The model under review builds one solid part; all positions refer to its coordinate system, in mm. Face numbers are marked on the shaded views. Round coordinates to 2 decimals unless told otherwise and drop trailing zeros. Order: outer loops, then holes, each group sorted by start corner. A loop starts at its lowest first (then second) coordinate and runs counter-clockwise, first axis right, second up. Notation, with made-up numbers: (22, 89.25) - (80, 89.25) arc R21 cw to (80, 106.25) - close; hole circle Ø7 at (4.5, 69.25). An arc over 180 degrees is marked (long way). One line per question, with ' | ' between items. Start each with the question number.
Item 1: For L1, parallel to X at y = 22, z = 5.25; L2, parallel to Y at x = -51, z = 15; L3, parallel to Z at x = -78.5, y = 29, list the stretches that pass through material, from the lowest coordinate up. Write a range as [from, to].
Item 2: Insertion check: pin 1 Ø2 at (x, y) = (-20.5, 15) entering from +Z. The pin has a flat end and moves straight along its axis. Give the tip position at first contact, or say it passes through.
Item 3: Draft analysis for pull direction X (two halves, no side actions). For the marked faces 1, 2, 3 and 4, state which applies: +X half, -X half, draft (parallel to the pull), parting line (faces both ways), or undercut.
Item 4: Add section B-B on x = -22.5. State the section outline as (y, z) points, and give its area (3 significant figures).
Item 5: Add section C-C on y = 22. State the section outline as (x, z) points, and give its area (3 significant figures).
Item 6: Add section A-A on z = 13.25. State the section outline as (x, y) points.
from build123d import *

# Parameters (mm, degrees)
F0_W     = 85.09
F0_H     = 44.958
F1_DEPTH = 29.6429
F2_R     = 3.048
F3_T     = -2.54


with BuildPart() as f1:
    # F0 (on Top) → F1 (new body)
    with BuildSketch(Plane.XY):
        with Locations((-42.545, 22.479)):
            Rectangle(F0_W, F0_H)
    extrude(amount=F1_DEPTH)

    # F2
    f2_edges = [f1.edges().sort_by_distance(p)[0] for p in [
        (-85.09, 44.958, 14.82145),
        (-85.09, 0, 14.82145),
        (0, 0, 14.82145),
        (0, 44.958, 14.82145),
    ]]
    fillet(f2_edges, radius=F2_R)

    # F3
    f3_openings = [f1.faces().sort_by_distance(p)[0] for p in [
        (-42.545, 22.479, 29.6429),
    ]]
    offset(amount=F3_T, openings=f3_openings)


solid = f1.part
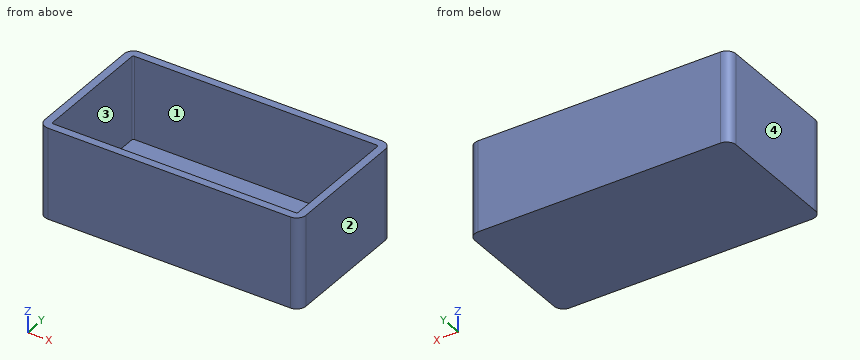
Determined:
1) L1: [-85.09, -82.55], [-2.54, 0] | L2: [0, 2.54], [42.42, 44.96] | L3: [0, 2.54]
2) pin 1: z = 2.54
3) face 1: undercut | face 2: +X half | face 3: undercut | face 4: -X half
4) outline: (0, 0) - (44.96, 0) - (44.96, 29.64) - (42.42, 29.64) - (42.42, 2.54) - (2.54, 2.54) - (2.54, 29.64) - (0, 29.64) - close | area: 252 mm2
5) outline: (-85.09, 0) - (0, 0) - (0, 29.64) - (-2.54, 29.64) - (-2.54, 2.54) - (-82.55, 2.54) - (-82.55, 29.64) - (-85.09, 29.64) - close | area: 354 mm2
6) outline: (-85.09, 3.05) arc R3.05 ccw to (-82.04, 0) - (-3.05, 0) arc R3.05 ccw to (0, 3.05) - (0, 41.91) arc R3.05 ccw to (-3.05, 44.96) - (-82.04, 44.96) arc R3.05 ccw to (-85.09, 41.91) - close; hole (-82.55, 3.05) arc R0.51 ccw to (-82.04, 2.54) - (-3.05, 2.54) arc R0.51 ccw to (-2.54, 3.05) - (-2.54, 41.91) arc R0.51 ccw to (-3.05, 42.42) - (-82.04, 42.42) arc R0.51 ccw to (-82.55, 41.91) - close
